from build123d import *

# Parameters (mm, degrees)
SKETCH_1_R      = 16.2
SKETCH_1_R_2    = 15.1
EXTRUDE_1_DEPTH = 2.5
SKETCH_3_R      = 1
FILLET_1_R      = 1


with BuildPart() as part:
    # 草图1 → 凸台-拉伸1 (new body, symmetric)
    with BuildSketch(Plane.XY):
        Circle(SKETCH_1_R)
        Circle(SKETCH_1_R_2, mode=Mode.SUBTRACT)
    extrude(amount=EXTRUDE_1_DEPTH, both=True)

    # 草图3 → 切除-旋转1 (revolve, cut)
    with BuildSketch(Plane(origin=(0, 0, 0), x_dir=(1, 0, 0), z_dir=(0, 1, 0))):
        with Locations((-14.6, 0)):
            Circle(SKETCH_3_R)
    revolve(axis=Axis((0, 0, 2.5), (0, 0, -1)), mode=Mode.SUBTRACT)

    # 圆角1
    fillet_1_edges = [part.edges().sort_by_distance(p)[0] for p in [
        (0, 15.1, 0.866025404),
        (0, -15.1, -0.866025404),
    ]]
    fillet(fillet_1_edges, radius=FILLET_1_R)


solid = part.part
Read the model definition and answer for the solid it produces. Units are mm, in the model's axes. Round coordinates to 2 decimals unless told otherwise and drop trailing zeros. Write each loop counter-clockwise with the first axis right and the second up, starting at its lowest first coordinate (ties: lowest second). Pieces come first, ordered by that corner, then holes.
1. The part is cut by section A-A, the plane z = 0.1. Determine the outline of the cut face in (x, y).
2. Given pin 1 Ø1.5 at (x, y) = (10, -7.5) entering from -Z; pin 2 Ø1.5 at (x, z) = (-4, -1.5) entering from +Y; pin 3 Ø1.5 at (x, z) = (7, 1) entering from -Y; pin 4 Ø2 at (x, z) = (9.5, 0) entering from +Y, each flat-ended and moving along its own axis, determine where each tip first touches the part or whether it passes through.
3. Determine the mould class of faces 1 (the face through (11, -11, -2.5)), 2 (the face through (-3.512, -15.815, 0.035)), 3 (the face through (-3.27, -14.74, 1.9)) for opening direction Y: pulls with the +Y half, pulls with the -Y half, needs draft (parallel to the pull), parting line crosses it, or undercut.
4. Straight lines are drawn through the part: L1, parallel to Y at x = 0, z = -1.8; L2, parallel to Y at x = -8, z = 0; L3, parallel to X at y = 8.5, z = -1.55. For each, find the intervals that lie inside material, in ascending order.
Values:
1. outline: circle Ø32.4 at (0, 0); hole circle Ø31.19 at (0, 0)
2. pin 1: passes through
2. pin 2: stops at y = 15.87
2. pin 3: stops at y = -14.95
2. pin 4: stops at y = 13.79
3. face 1: needs draft
3. face 2: parting line crosses it
3. face 3: undercut
4. L1: y = -16.2 to -15.1, 15.1 to 16.2
4. L2: y = -14.09 to -13.39, 13.39 to 14.09
4. L3: x = -13.79 to -12.48, 12.48 to 13.79
